from build123d import *


with BuildPart() as f2:
    # F2: sweep along a path in F0
    with BuildLine(Plane.YZ) as f2_path:
        Line((0, 0), (0, 50))
        ThreePointArc((0, 50), (25, 75), (50, 50))
        Line((50, 50), (50, 25))
        ThreePointArc((50, 25), (57.32233, 7.32233), (75, 0))
    # F1 (on Top) → F2 (sweep)
    with BuildSketch(Plane.XY):
        Polygon((6, -3.464102), (6, 3.464102), (0, 6.928203), (-6, 3.464102), (-6, -3.464102), (0, -6.928203), align=None)
    sweep(path=f2_path.line)


solid = f2.part
For this review, take the finished solid that the model builds, in its own axes (mm). A direction names the side the tool comes from. Round coordinates to 2 decimals unless told otherwise and drop trailing zeros. Write each loop counter-clockwise with the first axis right and the second up, starting at its lowest first coordinate (ties: lowest second). Pieces come first, ordered by that corner, then holes. Notation, with made-up numbers: (37.5, 31) - (61.5, 31) arc R15 ccw to (61.5, 50) - close; hole circle Ø7 at (65, -5). An arc over 180 degrees is marked (long way). Write item = value, one per line. Start each with the question number.
1. Consider section A-A on z = 48. State the section outline as (x, y) points.
2. Draft analysis for pull direction Y (two halves, no side actions). For faces 4 (the face through (2.96, -5.22, 25.35)), 5 (the face through (-0.4, 24.6, 68.3)), 6 (the face through (-5.625, 24.369, 78.674)), state which applies: released by +Y, released by -Y, zero draft, split by the parting line, or undercut.
3. For faces 1 (the face through (-3.042, 55.172, 37.325)), 2 (the face through (2.96, 55.22, 37.33)), 3 (the face through (0, 0, 0)), list the 3-axis set-ups (+Z, -Z, +X, -X, +Y, -Y) from which the entire face can be reached by the end or side of a thin tool; tool diameter is ignored.
4. Wall thickness on L1, parallel to Y at x = -4, z = 12; L2, parallel to Y at x = -2.75, z = 65.5; L3, parallel to X at y = 54, z = 45: over which ranges is each line inside the solid? List them lowest first.
5. Consider section D-D on x = -2.25. State the section outline as (y, z) points.
6. Consider section B-B on x = 3.75. State the section outline as (y, z) points, plus the area to 3 significant figures.
7. Consider section C-C on y = 25. State the section outline as (x, z) points, plus the area to 3 significant figures.
8. For pin 1 Ø4 at (x, y) = (0, 48.5) entering from -Z; pin 2 Ø6 at (x, z) = (1, 45) entering from +Y; pin 3 Ø2 at (x, z) = (3.5, 45.5) entering from -Y, all flat-tipped, find the tip position at first contact; note any pin that passes through.
Evaluation:
q1.outline = (-6, -3.46) - (0, -6.93) - (6, -3.46) - (6, 3.46) - (0, 6.93) - (-6, 3.46) - close; (-6, 46.54) - (0, 43.07) - (6, 46.54) - (6, 53.46) - (0, 56.93) - (-6, 53.46) - close
q2.face_4 = released by -Y
q2.face_5 = undercut
q2.face_6 = split by the parting line
q3.face_1 = +Z, -X, +Y
q3.face_2 = +Z, +X, +Y
q3.face_3 = -Z, +X, -X, -Y
q4.L1 = -4.62 to 4.62, 48.39 to 59.3
q4.L2 = -1.08 to 12.91, 37.09 to 51.08
q4.L3 = -5.07 to 5.07
q5.outline = (-5.63, 0) - (5.63, 0) - (5.63, 50) arc R19.37 cw to (44.37, 50) - (44.37, 25) arc R30.63 ccw to (75, -5.63) - (75, 5.63) arc R19.37 cw to (55.63, 25) - (55.63, 50) arc R30.63 ccw to (-5.63, 50) - close
q6.outline = (-4.76, 0) - (4.76, 0) - (4.76, 50) arc R20.24 cw to (45.24, 50) - (45.24, 25) arc R29.76 ccw to (75, -4.76) - (75, 4.76) arc R20.24 cw to (54.76, 25) - (54.76, 50) arc R29.76 ccw to (-4.76, 50) - close
q6.area = 1,840 mm2
q7.outline = (-6, 71.54) - (0, 68.07) - (6, 71.54) - (6, 78.46) - (0, 81.93) - (-6, 78.46) - close
q7.area = 125 mm2
q8.pin_1 = 4.53
q8.pin_2 = 56.93
q8.pin_3 = -5.48
